```python
from build123d import *

# Parameters (mm, degrees)
SKETCH_1_W          = 15
SKETCH_1_H          = 10.5
EXTRUDE_1_DEPTH     = 0.8
SKETCH_2_W          = 13
SKETCH_2_H          = 8.5
EXTRUDE_2_DEPTH     = 4.25
EXTRUDE_4_DEPTH     = 8.5
SKETCH_5_W          = 0.5
SKETCH_5_H          = 3.6
EXTRUDE_5_DEPTH     = 6.5
SKETCH_6_W          = 11
SKETCH_6_H          = 6.5
CUT_EXTRUDE_1_DEPTH = 1
EXTRUDE_6_DEPTH     = 3.15


with BuildPart() as part:
    # 草图1 → 凸台-拉伸1 (new body)
    with BuildSketch(Plane(origin=(0, 0, 0), x_dir=(1, 0, 0), z_dir=(0, 1, 0))):
        Rectangle(SKETCH_1_W, SKETCH_1_H)
    extrude(amount=EXTRUDE_1_DEPTH)

    # 草图2 → section 0 of loft_1
    with BuildSketch(Plane(origin=(0, -1.2, 0), x_dir=(-1, 0, 0), z_dir=(0, -1, 0)), mode=Mode.PRIVATE) as loft_1_s0:
        Rectangle(SKETCH_2_W, SKETCH_2_H)
    # loft up to a face of the part (loft_1)
    loft([loft_1_s0.sketch, part.faces().sort_by_distance((0, 0, 0))[0]])

    # 草图3 → 凸台-拉伸2 (add, symmetric)
    with BuildSketch(Plane.XY):
        Polygon((6.5, 9.8), (-6.5, 9.8), (-6.5, 6.8), (-6, 6.8), (-6, 0.8), (6, 0.8), (6, 6.8), (6.5, 6.8), align=None)
    extrude(amount=EXTRUDE_2_DEPTH, both=True)

    # 草图4 → 凸台-拉伸4 (add)
    with BuildSketch(Plane(origin=(0, 0, -4.25), x_dir=(-1, 0, 0), z_dir=(0, 0, -1))):
        Polygon((6.5, 6.8), (7.423732472, 3.591094946), (6.5, 0.8), (6, 0.8), (6.923732472, 3.591094946), (6, 6.8), align=None)
        Polygon((-6, 6.8), (-6.5, 6.8), (-7.423732472, 3.591094946), (-6.5, 0.8), (-6, 0.8), (-6.923732472, 3.591094946), align=None)
    extrude(amount=-EXTRUDE_4_DEPTH)

    # 草图5 → 凸台-拉伸5 (add)
    with BuildSketch(Plane(origin=(0, 9.8, 0), x_dir=(1, 0, 0), z_dir=(0, 1, 0))):
        Rectangle(SKETCH_5_W, SKETCH_5_H)
        with Locations((-5, 0)):
            Rectangle(SKETCH_5_W, SKETCH_5_H)
    extrude(amount=EXTRUDE_5_DEPTH)

    # 草图6 → 切除-拉伸1 (cut)
    with BuildSketch(Plane(origin=(0, -1.2, 0), x_dir=(-1, 0, 0), z_dir=(0, -1, 0))):
        Rectangle(SKETCH_6_W, SKETCH_6_H)
    extrude(amount=-CUT_EXTRUDE_1_DEPTH, mode=Mode.SUBTRACT)

    # 草图7 → 凸台-拉伸6 (add, symmetric)
    with BuildSketch(Plane.XY):
        with BuildLine():
            Line((-5.5, -0.2), (5.5, -0.2))
            Line((5.5, -0.2), (5.5, -1.2))
            ThreePointArc((5.5, -1.2), (1.062510248, -2.101360111), (-3.174011421, -3.7))
            ThreePointArc((-3.174011421, -3.7), (-4.635468683, -2.14834899), (-5.5, -0.2))
        make_face()
    extrude(amount=EXTRUDE_6_DEPTH, both=True)


solid = part.part
```
CAD build for the part. Positions are in the model's coordinates, mm. A direction names the side the tool comes from. Round coordinates to 2 decimals unless told otherwise and drop trailing zeros. Order: outer loops, then holes, each group sorted by start corner. A loop starts at its lowest first (then second) coordinate and runs counter-clockwise, first axis right, second up. Notation, with made-up numbers: (79, -22) -> (89, -22) arc R3 ccw to (89, -17) -> close; hole circle Ø9 at (32, 46). An arc over 180 degrees is marked (long way). Write item = value, one per line.
(1) Cut at B-B (y = 4.75). Write the cut outline in (x, z), plus the area to 4 significant figures.
Answers follow:
outline = (-7.09, -4.25) -> (-6.59, -4.25) -> (-6.59, 4.25) -> (-7.09, 4.25) -> close; (-6, -4.25) -> (6, -4.25) -> (6, 4.25) -> (-6, 4.25) -> close; (6.59, -4.25) -> (7.09, -4.25) -> (7.09, 4.25) -> (6.59, 4.25) -> close
area = 110.5 mm²
(2) Pull direction Y, two halves, no side cores. Call faces 4 (the cylindrical face through (1.124, -2.084, 0.044)), 5 (the flat face through (-6.47, 5.17, -0.06)), 6 (the flat face through (-0.25, 13, 0)): +Y half, -Y half, draft (parallel to the pull), parting line (faces both ways), or undercut.
Answers follow:
face_4 = -Y half
face_5 = undercut
face_6 = draft
(3) Cut at A-A (y = 12). Write the cut outline in (x, z).
Answers follow:
outline = (-5.25, -1.8) -> (-4.75, -1.8) -> (-4.75, 1.8) -> (-5.25, 1.8) -> close; (-0.25, -1.8) -> (0.25, -1.8) -> (0.25, 1.8) -> (-0.25, 1.8) -> close
(4) Drill centre lines: L1, parallel to X at y = 14.5, z = 0.5; L2, parallel to X at y = 5.75, z = -4; L3, parallel to X at y = 6, z = -1.25. Where is each one in solid material? Low to high.
Answers follow:
L1 = -5.25 to -4.75, -0.25 to 0.25
L2 = -6.8 to -6.3, -6 to 6, 6.3 to 6.8
L3 = -6.73 to -6.23, -6 to 6, 6.23 to 6.73
(5) 3-axis set-ups, long thin cutter, end or side, ignore diameter. For faces 1 (the flat face through (-6.97, 2.22, -0.06)), 2 (the flat face through (0.25, 13, 0)), 3 (the flat face through (0, 5, -4.25)): which of +Z, -Z, +X, -X, +Y, -Y reach the whole face in a straight line?
Answers follow:
face_1 = +Z, -Z, -X
face_2 = +Z, -Z, +X, +Y
face_3 = -Z, +X, -X, +Y
(6) Cut at C-C (z = 1.25). State how many separate pieces and enclosed holes the cut face has, plus the area to 3 significant figures.
Answers follow:
separate_pieces = 1
enclosed_holes = 2
area = 164 mm²
(7) Flat gauge pins, fed straight in: P1, Ø1.8, axis at y = 4, z = -2, coming from the +X side; P2, Ø3, axis at x = 2, y = 5, coming from the +Z side; P3, Ø2.5, axis at y = 9, z = -2, coming from the +X side. Where does each tip first touch, or does it go through?
Answers follow:
P1 = 7.42
P2 = 4.25
P3 = 6.5
